Design review of the part built by this model. Coordinates are the model's own, in mm. Round coordinates to 2 decimals unless told otherwise and drop trailing zeros. Write each loop counter-clockwise with the first axis right and the second up, starting at its lowest first coordinate (ties: lowest second). Pieces come first, ordered by that corner, then holes. Notation, with made-up numbers: (-0.5, 52.5) - (29.5, 52.5) arc R5 ccw to (29.5, 59.5) - close; hole circle Ø4 at (45.25, -4). An arc over 180 degrees is marked (long way). Use one line per item in the form item = value.
```python
from build123d import *

# Parameters (mm, degrees)
SKETCH1_R           = 0.85
BOSS_EXTRUDE1_DEPTH = 0.4


with BuildPart() as part:
    # Sketch1 → Boss-Extrude1 (new, symmetric)
    with BuildSketch(Plane(origin=(0, 0, 0), x_dir=(1, 0, 0), z_dir=(0, 1, 0))):
        with BuildLine():
            Line((-3.175, 6), (-3.175, 0))
            Line((-3.175, 0), (-4.1, 0))
            Line((-4.1, 0), (-4.1, -4.1))
            Line((-4.1, -4.1), (-3.125, -4.1))
            Line((-3.125, -4.1), (-3.125, -7.475))
            ThreePointArc((-3.125, -7.475), (-2.5, -8.1), (-1.875, -7.475))
            Line((-1.875, -7.475), (-1.875, -4.1))
            Line((-1.875, -4.1), (1.875, -4.1))
            Line((1.875, -4.1), (1.875, -7.475))
            ThreePointArc((1.875, -7.475), (2.5, -8.1), (3.125, -7.475))
            Line((3.125, -7.475), (3.125, -4.1))
            Line((3.125, -4.1), (4.1, -4.1))
            Line((4.1, -4.1), (4.1, 0))
            Line((4.1, 0), (3.175, 0))
            Line((3.175, 0), (3.175, 6))
            Line((3.175, 6), (1.875, 8))
            Line((1.875, 8), (-1.875, 8))
            Line((-1.875, 8), (-3.175, 6))
        make_face()
        with Locations(Location((0, 4, 0), (0, 0, 270))):
            Circle(SKETCH1_R, mode=Mode.SUBTRACT)
    extrude(amount=BOSS_EXTRUDE1_DEPTH, both=True)


solid = part.part
```
Q1. We need section B-B on y = 0.15. Write out the cut boundary in (x, z) (3 decimals).
Calculated:
outline = (-4.1, 0) - (-3.175, 0) - (-3.175, -6) - (-1.875, -8) - (1.875, -8) - (3.175, -6) - (3.175, 0) - (4.1, 0) - (4.1, 4.1) - (3.125, 4.1) - (3.125, 7.475) arc R0.625 ccw to (1.875, 7.475) - (1.875, 4.1) - (-1.875, 4.1) - (-1.875, 7.475) arc R0.625 ccw to (-3.125, 7.475) - (-3.125, 4.1) - (-4.1, 4.1) - close; hole circle Ø1.7 at (0, -4)
Q2. We need section C-C on z = -4. Write out the cut boundary in (x, y) (3 decimals), then the cut area to 3 significant figures.
Calculated:
outline = (-3.175, -0.4) - (-0.85, -0.4) - (-0.85, 0.4) - (-3.175, 0.4) - close; (0.85, -0.4) - (3.175, -0.4) - (3.175, 0.4) - (0.85, 0.4) - close
area = 3.72 mm2
Q3. To check wall thickness, follow line 1 along X through (y, z) = (0.3, 5.5) (3 decimals); line 2 along X through (y, z) = (0.1, -4) (3 decimals); line 3 along X through (y, z) = (-0.1, -2) (3 decimals). State the ranges of each line that lie inside material, in increasing order. Write a range as from..to.
Calculated:
line_1 = -3.125..-1.875, 1.875..3.125
line_2 = -3.175..-0.85, 0.85..3.175
line_3 = -3.175..3.175
Q4. We need section D-D on x = -1.5. Write out the cut boundary in (y, z).
Calculated:
outline = (-0.4, -8) - (0.4, -8) - (0.4, 4.1) - (-0.4, 4.1) - close
Q5. For P1, Ø1.4, axis at x = 0, z = -4, coming from the +Y side, flat-tipped, find the tip position at first contact; note if it passes through.
Calculated:
P1 = through
Q6. Draft analysis for pull direction X (two halves, no side actions). For faces 1 (the cylindrical face through (-0.52, -0.01, -4.67)), 2 (the flat face through (0, 0.4, 0)), 3 (the flat face through (-2.52, 0.01, -7.01)), state which applies: released by +X, released by -X, zero draft, split by the parting line, or undercut.
Calculated:
face_1 = undercut
face_2 = zero draft
face_3 = released by -X
Q7. We need section A-A on x = 0. Write out the cut boundary in (y, z), then the cut area to 3 significant figures.
Calculated:
outline = (-0.4, -8) - (0.4, -8) - (0.4, -4.85) - (-0.4, -4.85) - close; (-0.4, -3.15) - (0.4, -3.15) - (0.4, 4.1) - (-0.4, 4.1) - close
area = 8.32 mm2
